For this review, take the finished solid that the model builds, in its own axes (mm). Face numbers are marked on the shaded views. A direction names the side the tool comes from. Coordinates: 2 decimals unless noted, no trailing zeros. Order: outer loops, then holes, each group sorted by start corner. A loop starts at its lowest first (then second) coordinate and runs counter-clockwise, first axis right, second up.
from build123d import *

# Parameters (mm, degrees)
F1_DEPTH = 10
F2_W     = 8
F2_H     = 50
F3_DEPTH = 24
F4_W     = 10
F4_H     = 50
F5_DEPTH = 70
F6_R     = 18
F6_R_2   = 12
F7_DEPTH = 15
F8_R     = 12
F9_DEPTH = 10


with BuildPart() as f1:
    # F0 (on Top) → F1 (new body)
    with BuildSketch(Plane.XY):
        with BuildLine():
            Line((0, 50), (0, 0))
            Line((0, 0), (63, 0))
            ThreePointArc((63, 0), (88, 25), (63, 50))
            Line((63, 50), (0, 50))
        make_face()
        with BuildLine():
            ThreePointArc((78, 25), (73.606602, 14.393398), (63, 10))
            ThreePointArc((63, 10), (48, 25), (63, 40))
            ThreePointArc((63, 40), (73.606602, 35.606602), (78, 25))
        make_face(mode=Mode.SUBTRACT)
    extrude(amount=F1_DEPTH)

    # F2 (on face) → F3 (join)
    with BuildSketch(Plane.XY.offset(10)):
        with Locations((34, 25)):
            Rectangle(F2_W, F2_H)
    extrude(amount=F3_DEPTH)

    # F4 (on face) → F5 (join)
    with BuildSketch(Plane.XY.offset(10)):
        with Locations((5, 25)):
            Rectangle(F4_W, F4_H)
    extrude(amount=F5_DEPTH)

    # F6 (on face) → F7 (join)
    with BuildSketch(Plane.YZ.offset(10)):
        with Locations((25, 56)):
            Circle(F6_R)
        with Locations((25, 56)):
            Circle(F6_R_2, mode=Mode.SUBTRACT)
    extrude(amount=F7_DEPTH)

    # F8 (on face) → F9 (cut, through all)
    with BuildSketch(Plane.YZ.offset(10)):
        with Locations((25, 56)):
            Circle(F8_R)
    extrude(amount=-F9_DEPTH, mode=Mode.SUBTRACT)


solid = f1.part
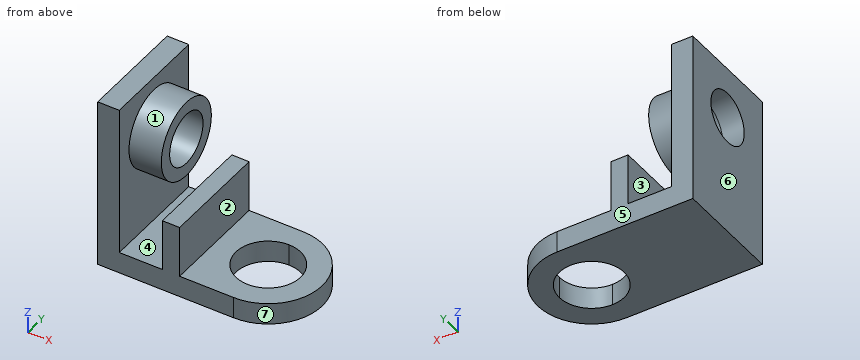
1. Take a section at D-D, the plane z = 6. Give the boundary of the cut face in (x, y), plus the area to 3 significant figures.
Answer below:
outline: (0, 0) - (63, 0) arc R25 ccw to (63, 50) - (0, 50) - close; hole (63, 40) arc R15 ccw (long way) to (78, 25) arc R15 ccw to start
area: 3,420 mm2
2. Clearance check with flat-ended pins moving along their axes: pin 1 Ø8 at (y, z) = (23, 48.5) entering from -X; pin 2 Ø6 at (x, y) = (16, 19) entering from +Z; pin 3 Ø25 at (y, z) = (26.5, 30.5) entering from +X; pin 4 Ø3 at (x, y) = (32.5, 30) entering from +Z. State where each tip first meets the part, or that it passes through.
Answer below:
pin 1: passes through
pin 2: stops at z = 73.75
pin 3: stops at x = 38
pin 4: stops at z = 34
3. Take a section at B-B, the plane z = 56. Give the boundary of the cut face in (x, y).
Answer below:
outline: (0, 0) - (10, 0) - (10, 7) - (25, 7) - (25, 13) - (0, 13) - close; (0, 37) - (25, 37) - (25, 43) - (10, 43) - (10, 50) - (0, 50) - close
4. Take a section at C-C, the plane y = 27. Give the boundary of the cut face in (x, z).
Answer below:
outline: (0, 0) - (48.13, 0) - (48.13, 10) - (38, 10) - (38, 34) - (30, 34) - (30, 10) - (10, 10) - (10, 38.11) - (25, 38.11) - (25, 44.17) - (0, 44.17) - close; (0, 67.83) - (25, 67.83) - (25, 73.89) - (10, 73.89) - (10, 80) - (0, 80) - close; (77.87, 0) - (87.92, 0) - (87.92, 10) - (77.87, 10) - close
5. To check wall thickness, follow L1, parallel to X at y = 41, z = 18.5; L2, parallel to Z at x = 11, y = 24; L3, parallel to Z at x = 7, y = 25. State the ranges of each line that lie inside material, in increasing order.
Answer below:
L1: x = 0 to 10, 30 to 38
L2: z = 0 to 10, 38.03 to 44.04, 67.96 to 73.97
L3: z = 0 to 44, 68 to 80
6. Take a section at A-A, the plane x = 15. Give the boundary of the cut face in (y, z), plus the area to 3 significant figures.
Answer below:
outline: (0, 0) - (50, 0) - (50, 10) - (0, 10) - close; circle Ø36 at (25, 56); hole circle Ø24 at (25, 56)
area: 1,070 mm2
7. Machinability: for the marked faces 1, 2 and 3, which of the approach directions +Z, -Z, +X, -X, +Y, -Y give a long, thin tool a straight path to every point of the face, cutting with its end or side? Answer none if there is none.
Answer below:
face 1: +X
face 2: +Z, +X, +Y, -Y
face 3: +Z, +Y, -Y
8. The part is to be moulded in two halves that separate along X. For the marked faces 4, 5, 6 and 7, say which applies: +X half, -X half, draft (parallel to the pull), parting line (faces both ways), or undercut.
Answer below:
face 4: undercut
face 5: draft
face 6: -X half
face 7: +X half
